from build123d import *

# Parameters (mm, degrees)
SKETCH_1_W          = 13.5
SKETCH_1_H          = 11
EXTRUDE_1_DEPTH     = 1.6
SKETCH_2_W          = 7.5
SKETCH_2_H          = 9.5
EXTRUDE_2_DEPTH     = 9.5
SKETCH_3_W          = 7.180285824
SKETCH_3_H          = 10.458318516
EXTRUDE_3_DEPTH     = 6
SKETCH_4_W          = 6.139304191
SKETCH_4_H          = 9.400260038
CUT_EXTRUDE_1_DEPTH = 6
SKETCH_5_R          = 3.05
EXTRUDE_4_DEPTH     = 13


with BuildPart() as part:
    # 草图1 → 凸台-拉伸1 (new body)
    with BuildSketch(Plane(origin=(0, 0, 0), x_dir=(1, 0, 0), z_dir=(0, 1, 0))):
        with Locations((-6.339102869, 0.04845815)):
            Rectangle(SKETCH_1_W, SKETCH_1_H)
    extrude(amount=EXTRUDE_1_DEPTH)

    # 草图2 → 凸台-拉伸2 (add)
    with BuildSketch(Plane(origin=(0, 1.6, 0), x_dir=(1, 0, 0), z_dir=(0, 1, 0))):
        with Locations((-11.339102869, 0.04845815)):
            Rectangle(SKETCH_2_W, SKETCH_2_H)
    extrude(amount=EXTRUDE_2_DEPTH)

    # 草图3 → 凸台-拉伸3 (add)
    with BuildSketch(Plane(origin=(0, 1.6, 0), x_dir=(1, 0, 0), z_dir=(0, 1, 0))):
        with Locations((-3.428185131, -0.064528037)):
            Rectangle(SKETCH_3_W, SKETCH_3_H)
    extrude(amount=EXTRUDE_3_DEPTH)

    # 草图4 → 切除-拉伸1 (cut)
    with BuildSketch(Plane(origin=(0, 7.6, 0), x_dir=(1, 0, 0), z_dir=(0, 1, 0))):
        with Locations((-3.408558638, -0.075891751)):
            Rectangle(SKETCH_4_W, SKETCH_4_H)
    extrude(amount=-CUT_EXTRUDE_1_DEPTH, mode=Mode.SUBTRACT)

    # 草图5 → 凸台-拉伸4 (add)
    with BuildSketch(Plane.ZY.offset(15.089102869)):
        with Locations(Location((0, 6.221255945, 0), (0, 0, 180))):
            Circle(SKETCH_5_R)
    extrude(amount=EXTRUDE_4_DEPTH)


solid = part.part
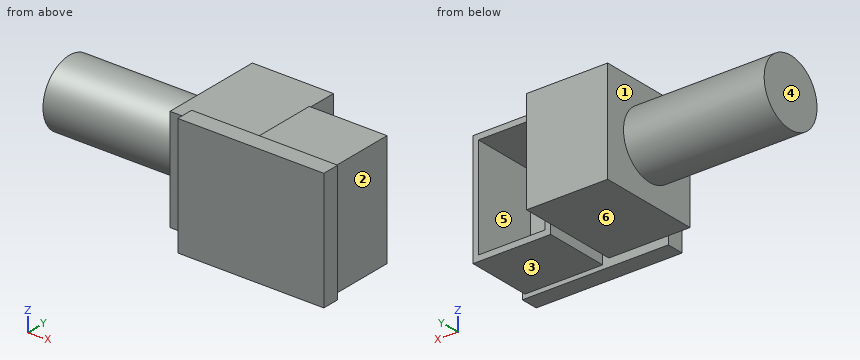
The listing builds one solid part. Answer for the finished solid, in the listing's coordinates (mm). Face numbers are marked on the shaded views. A direction names the side the tool comes from. Give positions to 0.01 mm unless a question says otherwise; leave off trailing zeros. Write each loop counter-clockwise with the first axis right and the second up, starting at its lowest first coordinate (ties: lowest second). Pieces come first, ordered by that corner, then holes.
Item 1: Section A-A, the plane y = 6.75 is taken. Write down the section's boundary in (x, z).
Item 2: Section D-D, the plane y = 10 is taken. Write down the section's boundary in (x, z).
Item 3: Flat-ended cylindrical pins translate along their axes: P1, Ø5, axis at x = -2.5, y = 6, coming from the +Z side; P2, Ø1.8, axis at x = -5, z = -2, coming from the +Y side; P3, Ø3, axis at x = -5, y = 5, coming from the -Z side; P4, Ø5, axis at y = 4, z = -1.5, coming from the +X side. Find the tip coordinate at first contact, or state that the pin passes through.
Item 4: Which of the six approach directions +Z, -Z, +X, -X, +Y, -Y give full straight-line access (tool end or side, diameter ignored) to the marked faces 1, 2 and 3?
Item 5: Determine the mould class of the marked faces 4, 5 and 6 for opening direction Z: released by +Z, released by -Z, zero draft, split by the parting line, or undercut.
Item 6: Find the intervals of material crossed by line 1 along X through (y, z) = (3, 1.5); line 2 along X through (y, z) = (3.5, -0.75); line 3 along X through (y, z) = (10, 3), in increasing order.
Item 7: Section C-C, the plane x = -9 is taken. Write down the section's boundary in (y, z), plus the area to 3 significant figures.
Item 8: Section B-B, the plane z = 0 is taken. Write down the section's boundary in (x, y), plus the area to 3 significant figures.
Completed:
1. outline: (-28.09, -3) - (-15.09, -3) - (-15.09, -4.8) - (-7.59, -4.8) - (-7.59, 4.7) - (-15.09, 4.7) - (-15.09, 3) - (-28.09, 3) - close; (-7.02, -5.16) - (0.16, -5.16) - (0.16, 5.29) - (-7.02, 5.29) - close; hole (-6.48, -4.62) - (-0.34, -4.62) - (-0.34, 4.78) - (-6.48, 4.78) - close
2. outline: (-15.09, -4.8) - (-7.59, -4.8) - (-7.59, 4.7) - (-15.09, 4.7) - close
3. P1: stops at z = 5.29
3. P2: stops at y = 1.6
3. P3: stops at z = -5.16
3. P4: stops at x = 0.41
4. face 1: -X
4. face 2: +Z, -Z, +X, +Y
4. face 3: -Z, +X, -X, +Y
5. face 4: zero draft
5. face 5: undercut
5. face 6: released by -Z
6. line 1: x = -15.09 to -7.59, -7.02 to -6.48, -0.34 to 0.16
6. line 2: x = -28.09 to -7.59, -7.02 to -6.48, -0.34 to 0.16
6. line 3: x = -15.09 to -7.59
7. outline: (0, -5.55) - (1.6, -5.55) - (1.6, -4.8) - (11.1, -4.8) - (11.1, 4.7) - (1.6, 4.7) - (1.6, 5.45) - (0, 5.45) - close
7. area: 108 mm2
8. outline: (-28.09, 3.17) - (-15.09, 3.17) - (-15.09, 1.6) - (-13.09, 1.6) - (-13.09, 0) - (0.41, 0) - (0.41, 1.6) - (0.16, 1.6) - (0.16, 7.6) - (-0.34, 7.6) - (-0.34, 1.6) - (-6.48, 1.6) - (-6.48, 7.6) - (-7.02, 7.6) - (-7.02, 1.6) - (-7.59, 1.6) - (-7.59, 11.1) - (-15.09, 11.1) - (-15.09, 9.27) - (-28.09, 9.27) - close
8. area: 178 mm2
